Verification items for the finished model (mm, model axes). A direction names the side the tool comes from. Coordinates: 2 decimals unless noted, no trailing zeros. Loops run counter-clockwise (first coordinate to the right, second up) from the corner with the lowest first, then second, coordinate; pieces in that order, holes last. Notation, with made-up numbers: (18.25, -25.75) -> (40.25, -25.75) arc R19 ccw to (40.25, 2.25) -> close; hole circle Ø10 at (-12, 69). An arc over 180 degrees is marked (long way). Answer as a JSON object with one key per item and string values. Group by question number.
Q1. Cross-section at A-A on z = 0. Record the boundary of the cut face in (x, y), and give its area (3 significant figures).
Q2. Cross-section at D-D on y = 13. Give the number of separate pieces and of enclosed holes in the cut face, and give its area (3 significant figures).
Q3. Release check for a two-part mould opening along Z. For faces 3 (the cylindrical face through (-4.54, 15.2, -15.52)), 4 (the cylindrical face through (-4.51, 30.88, 0.21)), 5 (the cylindrical face through (-0.76, 15.4, -8.3)) record: released by +Z, released by -Z, zero draft, split by the parting line, or undercut.
Q4. Scan lines: L1, parallel to Y at x = 1.5, z = 0; L2, parallel to Z at x = -0.5, y = 12.5; L3, parallel to Z at x = 0, y = 17.5. Record each from-to range of solid material in increasing order.
Q5. Cross-section at B-B on y = 4. Record the boundary of the cut face in (x, z) (1 decimal), and give its area (3 significant figures).
Q6. Set-up check for faces 1 (the cylindrical face through (-0.954, 27.894, -0.833)), 2 (the cylindrical face through (-0.027, 22.345, 0.883)): record each of +Z, -Z, +X, -X, +Y, -Y from which the full face is reachable in a straight line by a thin tool's end or side.
Q7. Gauge pin test, flat ends, axial feed: pin 1 Ø1 at (y, z) = (19.5, 3) entering from -X; pin 2 Ø2 at (x, z) = (-0.19, 0) entering from +Y. Record the tip position at first contact, or that the pin passes through.
Q8. Cross-section at C-C on x = 4. Record the boundary of the cut face in (y, z), and give its area (3 significant figures).
Autodesk Inventor part; units mm, degrees
ref_plane "YZ Plane" through (0, 0, 0) normal (1, 0, 0) x (0, 1, 0)
ref_plane "XZ Plane" through (0, 0, 0) normal (0, 1, 0) x (-1, 0, 0)
ref_plane "XY Plane" through (0, 0, 0) normal (0, 0, 1) x (1, 0, 0)
sketch "Sketch1" plane through (0, 0, 0) normal (0, 1, 0) x (-1, 0, 0)
  line L0 (-4.7371, 18.5916) -> (-4.7371, -18.5916)
  line L1 (4.8895, -15.875) -> (4.8895, 15.875)
  circle A0 centre (4.8895, -34.29) radius 18.415
  circle A1 centre (4.8895, 34.29) radius 18.415
  point P0 (0, 0)
  point P1 (4.8895, 0)
  dimension "d3" = 31.75
  dimension "d10" = 36.83
  dimension "d11" = 9.6266
  dimension "d12" = 4.8895
  dimension "d13" = 0
  dimension "d14" = 0
  dimension "d15" = 16.6109
extrude "Extrusion1" add sketch "Sketch1" along normal blind 31.242 contours A1 L1 A0 L0
sketch "Sketch2" plane through (4.7371, 0, 18.5916) normal (1, 0, 0) x (0, 0, -1)
  circle A0 centre (18.5916, 15.621) radius 6.7818
  line L0 (0, 31.242) -> (37.1831, 31.242)
  line L1 (0, 0) -> (0, 31.242)
  point P0 (18.5916, 0)
  point P1 (18.5916, 31.242)
  point P2 (0, 15.621)
  dimension "d39" = 13.5636
extrude "Extrusion2" cut sketch "Sketch2" against normal through all
fillet "Fillet1" radius 1.27 10 edges at (4.7371, 15.621, 6.7818) (-4.8895, 15.621, 6.7818) (4.7371, 31.242, 0) (4.7371, 15.621, -18.5916) (4.7371, 15.621, 18.5916) (-4.8895, 15.621, 15.875) (0.1118, 31.242, 16.5671) (0.1118, 31.242, -16.5671) (-4.8895, 31.242, 0) (-4.8895, 15.621, -15.875)
sketch "Sketch3" plane through (0, 31.242, 0) normal (0, 1, 0) x (1, 0, 0)
  arc A0 (2.928, -17.6167) -> (4.7371, -16.4668) centre (3.4671, -16.4668) ccw
  arc A1 (4.7371, 16.4668) -> (2.928, 17.6167) centre (3.4671, 16.4668) ccw
  line L0 (-4.8895, 14.646) -> (-4.8895, -14.646)
  point P0 (0, 0)
  point P1 (-0.1905, -10.1168)
  point P2 (-0.1905, 10.1168)
  dimension "d22" = 6.35
  dimension "d23" = 6.35
  dimension "d38" = 4.699
hole "Hole1" at (-0.1905, 31.242, 10.1168) at (-0.1905, 31.242, -10.1168) direction (0, -1, 0) diameter 3.81 end through all
sketch "Sketch4" plane through (0, 31.242, 0) normal (0, 1, 0) x (1, 0, 0)
  circle A0 centre (-0.1905, -10.1168) radius 1.905
  circle A1 centre (-0.1905, 10.1168) radius 1.905
  arc A2 (-3.6195, 14.646) -> (3.4671, 16.4668) centre (-4.8895, 34.29) ccw
  line L0 (-3.6195, -14.646) -> (-3.6195, 14.646)
  arc A3 (3.4671, -16.4668) -> (-3.6195, -14.646) centre (-4.8895, -34.29) ccw
  line L1 (3.4671, 16.4668) -> (3.4671, -16.4668)
  point P0 (0, 0)
  point P1 (-0.1905, 0)
hole "Hole2" at (-0.1905, 31.242, 0) direction (0, -1, 0) diameter 2.2606 depth 6.604
properties part number "BatteryBrace"
Computed values:
{
 "1": {"outline": "(-4.89, 0) -> (4.74, 0) -> (4.74, 7.57) arc R1.27 ccw to (3.47, 8.84) -> (-3.62, 8.84) arc R1.27 ccw to (-4.89, 7.57) -> close; (-4.89, 23.67) arc R1.27 ccw to (-3.62, 22.4) -> (3.47, 22.4) arc R1.27 ccw to (4.74, 23.67) -> (4.74, 29.97) arc R1.27 ccw to (3.47, 31.24) -> (0.94, 31.24) -> (0.94, 24.64) -> (-1.32, 24.64) -> (-1.32, 31.24) -> (-3.62, 31.24) arc R1.27 ccw to (-4.89, 29.97) -> close", "area": "153 mm²"},
 "2": {"separate pieces": "2", "enclosed holes": "2", "area": "175 mm²"},
 "3": {"face 3": "released by -Z", "face 4": "zero draft", "face 5": "undercut"},
 "4": {"L1": "y = 0 to 8.84, 22.4 to 31.24", "L2": "z = -16.41 to -12, -8.24 to -6.02, 6.02 to 8.24, 12 to 16.41", "L3": "z = -16.54 to -12.01, -8.22 to -6.52, 6.52 to 8.22, 12.01 to 16.54"},
 "5": {"outline": "(-4.9, -14.6) arc R1.3 ccw to (-3.7, -15.9) arc R18.4 cw to (2.9, -17.6) arc R1.3 ccw to (4.7, -16.5) -> (4.7, 16.5) arc R1.3 ccw to (2.9, 17.6) arc R18.4 cw to (-3.7, 15.9) arc R1.3 ccw to (-4.9, 14.6) -> close; hole circle Ø3.8 at (-0.2, -10.1); hole circle Ø3.8 at (-0.2, 10.1)", "area": "297 mm²"},
 "6": {"face 1": "+Y", "face 2": "+X, -X"},
 "7": {"pin 1": "passes through", "pin 2": "stops at y = 24.64"},
 "8": {"outline": "(0, -17.62) -> (29.97, -17.62) arc R1.15 ccw to (31.12, -16.47) -> (31.12, 16.47) arc R1.15 ccw to (29.97, 17.62) -> (0, 17.62) -> close; hole circle Ø13.8 at (15.62, 0)", "area": "947 mm²"}
}
